Autodesk Inventor part; units mm, degrees
ref_plane "Work Plane1" through (3.837, 85.8, -2.502) normal (-1, 0, 0) x (0, -1, 0)
ref_plane "YZ Plane" through (0, 0, 0) normal (1, 0, 0) x (0, 1, 0)
ref_plane "XZ Plane" through (0, 0, 0) normal (0, 1, 0) x (-1, 0, 0)
sketch "Sketch1" plane through (0, 0, 0) normal (0, 1, 0) x (-1, 0, 0)
  arc A0 (-1.337, 0) -> (0, -5.9706) centre (12.663, 0) ccw
  line L0 (-1.337, 0) -> (0, 0)
  line L1 (0, -5.9706) -> (-2.6226, -6.213)
  line L2 (0, -5.9706) -> (5.1195, -5.9706) construction
  line L3 (0, 5.9706) -> (-2.6226, 6.213)
  line L4 (0, 5.9706) -> (2.6337, 5.9706) construction
  arc A1 (0, 5.9706) -> (-1.337, 0) centre (12.663, 0) ccw
  line L5 (-3.6462, -2.502) -> (-3.837, -2.502)
  line L6 (-3.6462, 2.502) -> (-3.837, 2.502)
  line L7 (-3.837, -2.502) -> (-8.337, -2.502)
  line L8 (-8.337, -2.502) -> (-8.337, 2.502)
  line L9 (-8.337, 2.502) -> (-3.837, 2.502)
  arc A2 (-2.6226, 6.213) -> (-3.6462, 2.502) centre (12.663, 0) ccw
  arc A3 (-3.6462, -2.502) -> (-2.6226, -6.213) centre (12.663, 0) ccw
  dimension "d2" = 174.72
  dimension "d3" = 174.72
  dimension "d7" = 4.5
extrude "Extrusion1" add sketch "Sketch1" along normal blind 85.8
fillet "Fillet1" radius 4.5 2 edges at (8.337, 85.8, 0) (8.337, 0, 0)
ref_plane "Work Plane1" through (3.837, 85.8, -2.502) normal (-1, 0, 0) x (0, -1, 0)
sketch "Sketch2" plane through (3.837, 85.8, -2.502) normal (-1, 0, 0) x (0, -1, 0)
  line L0 (0, 0) -> (0, 5.004)
  line L1 (0, 2.502) -> (15, 2.502) construction
  line L2 (85.8, 5.004) -> (85.8, 0)
  line L3 (85.8, 2.502) -> (70.8, 2.502) construction
  circle A0 centre (15, 2.502) radius 1.5
  line L4 (70.8, 2.502) -> (70.9, 2.502) construction
  circle A1 centre (70.9, 2.502) radius 1.5
  line L5 (70.9, 2.502) -> (71.1, 2.502) construction
  line L6 (71.1, 2.502) -> (71.1, 4.6181) construction
  dimension "d11" = 15
  dimension "d13" = 3
  dimension "d23" = 0.2
extrude "Extrusion2" cut sketch "Sketch2" along normal blind 7 contours A0
extrude "Extrusion3" cut sketch "Sketch2" along normal up to surface contours A1
properties part number "Grip"
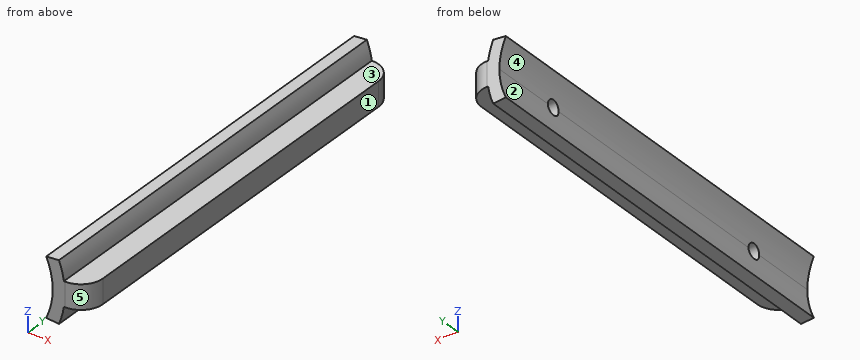
Input: part model. Units: mm. Frame: model coordinates. Face numbers are marked on the shaded views. A direction names the side the tool comes from. Coordinates: 2 decimals unless noted, no trailing zeros. Write each loop counter-clockwise with the first axis right and the second up, starting at its lowest first coordinate (ties: lowest second). Pieces come first, ordered by that corner, then holes. Notation, with made-up numbers: M 69,-36.75 L 76,-36.75 A22 cw 76,-21.75 Z; hole C 56.5,-24 d1. An arc over 180 degrees is marked long. Answer as a JSON object with one key per item and string values. Group by question number.
(1) Set-up query: the marked faces 1 and 2. Return all of +Z, -Z, +X, -X, +Y, -Y with unobstructed straight access to the full face (end or side cutting, diameter ignored); none if empty.
(2) Section B-B on z = 3.5. Output: boundary loops of the cut face in (x, y), plus the area to 3 significant figures.
(3) Section C-C on x = 7.5. Output: boundary loops of the cut face in (y, z), plus the area to 3 significant figures.
(4) Contact query for flat-ended pins moving along their axis: P1, Ø1, axis at y = 21.5, z = -4, coming from the +X side; P2, Ø2.5, axis at y = 14.9, z = 0, coming from the -X side; P3, Ø2.5, axis at y = 71, z = 0.5, coming from the -X side. Output: stop coordinate, or through.
(5) Section D-D on y = 14.9. Output: boundary loops of the cut face in (x, z).
(6) Section A-A on y = 55.5. Output: boundary loops of the cut face in (x, z).
(7) Ray query, line 1 along Y through (x, z) = (2.15, 0); line 2 along Z through (x, y) = (7.25, 66.5); line 3 along X through (y, z) = (8, 1.5). Return the intervals inside material, ascending. Write a range as [from, to].
(8) Mould query, pull axis Z, two halves, no side actions, for the marked faces 3, 4 and 5. Classes: pulls with the +Z half, pulls with the -Z half, needs draft (parallel to the pull), parting line crosses it, or undercut.
Result set:
{
 "1": {"face 1": "+Z, -Z, +X, +Y, -Y", "face 2": "-X, +Y, -Y"},
 "2": {"outline": "M 0.89,0 L 3.46,0 L 3.46,85.8 L 0.89,85.8 Z", "area": "220 mm2"},
 "3": {"outline": "M 1.89,-2.5 L 83.91,-2.5 L 83.91,2.5 L 1.89,2.5 Z", "area": "410 mm2"},
 "4": {"P1": "stops at x = 3.46", "P2": "stops at x = 3.84", "P3": "stops at x = 1.23"},
 "5": {"outline": "M 0,-5.97 L 2.62,-6.21 A16.5 ccw 3.65,-2.5 L 8.34,-2.5 L 8.34,2.5 L 3.65,2.5 A16.5 ccw 2.62,6.21 L 0,5.97 A14 cw 1.26,1.5 L 3.84,1.5 L 3.84,-1.5 L 1.26,-1.5 A14 cw Z"},
 "6": {"outline": "M 0,-5.97 L 2.62,-6.21 A16.5 ccw 3.65,-2.5 L 8.34,-2.5 L 8.34,2.5 L 3.65,2.5 A16.5 ccw 2.62,6.21 L 0,5.97 A14 cw 1.34,0 A14 cw Z"},
 "7": {"line 1": "y = [0, 13.4], [16.4, 69.3], [72.3, 85.8]", "line 2": "z = [-2.5, 2.5]", "line 3": "x = [1.26, 8.34]"},
 "8": {"face 3": "pulls with the +Z half", "face 4": "undercut", "face 5": "needs draft"}
}
